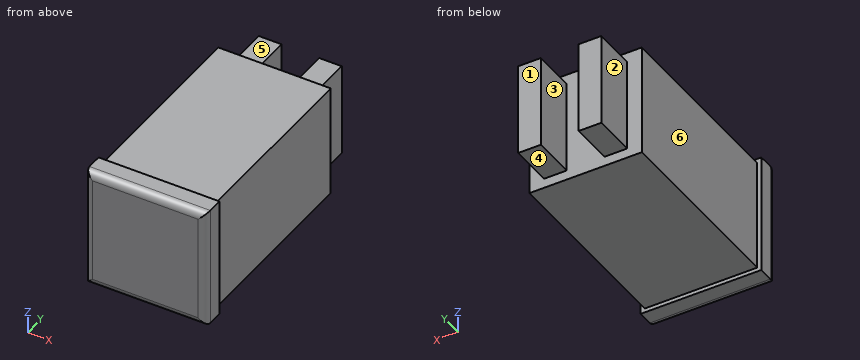
from build123d import *

# Parameters (mm, degrees)
F0_W     = 44.7
F0_H     = 44.7
F0_W_2   = 40.7
F0_H_2   = 40.7
F1_DEPTH = 73
F2_W     = 44.7
F2_H     = 44.7
F2_W_2   = 40.7
F2_H_2   = 40.7
F2_W_3   = 9
F2_H_3   = 37
F3_DEPTH = 3
F4_DEPTH = 20
F0_W_3   = 48
F0_H_3   = 48
F5_DEPTH = 9
F6_R     = 3


with BuildPart() as f1:
    # F0 (on Front) → F1 (new body)
    with BuildSketch(Plane.XZ):
        Rectangle(F0_W, F0_H)
        Rectangle(F0_W_2, F0_H_2, mode=Mode.SUBTRACT)
    extrude(amount=-F1_DEPTH)

    # F2 (on face) → F3 (join)
    with BuildSketch(Plane(origin=(0, 73, 0), x_dir=(-1, 0, 0), z_dir=(0, 1, 0))):
        Rectangle(F2_W, F2_H)
        Rectangle(F2_W_2, F2_H_2, mode=Mode.SUBTRACT)
        Rectangle(F2_W_2, F2_H_2)
        with Locations((-12, 0)):
            Rectangle(F2_W_3, F2_H_3, mode=Mode.SUBTRACT)
        with Locations((12, 0)):
            Rectangle(F2_W_3, F2_H_3, mode=Mode.SUBTRACT)
    extrude(amount=F3_DEPTH)

    # F2 (on face) → F4 (join)
    with BuildSketch(Plane(origin=(0, 73, 0), x_dir=(-1, 0, 0), z_dir=(0, 1, 0))):
        with Locations((-12, 0)):
            Rectangle(F2_W_3, F2_H_3)
        with Locations((12, 0)):
            Rectangle(F2_W_3, F2_H_3)
    extrude(amount=F4_DEPTH)

    # F0 (on Front) → F5 (join)
    with BuildSketch(Plane.XZ):
        Rectangle(F0_W_3, F0_H_3)
        Rectangle(F0_W, F0_H, mode=Mode.SUBTRACT)
        Rectangle(F0_W, F0_H)
        Rectangle(F0_W_2, F0_H_2, mode=Mode.SUBTRACT)
        Rectangle(F0_W_2, F0_H_2)
    extrude(amount=F5_DEPTH)

    # F6
    f6_edges = [f1.edges().sort_by_distance(p)[0] for p in [
        (24, -9, 0),
        (0, -9, 24),
        (-24, -9, 0),
        (0, -9, -24),
    ]]
    fillet(f6_edges, radius=F6_R)


solid = f1.part
Geometry check sheet. Reference: the model listing, model coordinates, mm. Face numbers are marked on the shaded views. A direction names the side the tool comes from. Round coordinates to 2 decimals unless told otherwise and drop trailing zeros. Loops run counter-clockwise (first coordinate to the right, second up) from the corner with the lowest first, then second, coordinate; pieces in that order, holes last. Notation, with made-up numbers: (-35.5, -18.5) -> (19.5, -18.5) arc R23 cw to (19.5, -10.5) -> close; hole circle Ø1 at (-11.5, 66.25). An arc over 180 degrees is marked (long way). Answer as a JSON object with one key per item and string values. Group by question number.
Item 1: Cross-section at A-A, the plane x = -5.5. Record the cut outline in (y, z).
Item 2: Cross-section at B-B, the plane z = -16. Record the cut outline in (x, y), plus the area to 3 significant figures.
Item 3: Set-up check for the marked faces 4, 5 and 6: record each of +Z, -Z, +X, -X, +Y, -Y from which the full face is reachable in a straight line by a thin tool's end or side.
Item 4: Release check for a two-part mould opening along X. For the marked faces 1, 2 and 3 record: pulls with the +X half, pulls with the -X half, needs draft (parallel to the pull), parting line crosses it, or undercut.
Item 5: Cross-section at C-C, the plane y = 26.5. Record the cut outline in (x, z).
Item 6: Thickness scan on line 1 along Y through (x, z) = (-8.5, 4); line 2 along Z through (x, y) = (3, 38). Record the ranges inside material, lowest first.
Item 7: Cross-section at D-D, the plane x = -13.5. Record the cut outline in (y, z), plus the area to 3 significant figures.
Item 8: Depth check by flat-ended pin: pin 1 Ø8 at (x, y) = (16.5, 51) entering from +Z; pin 2 Ø22.5 at (y, z) = (20.5, -9) entering from +X; pin 3 Ø20.5 at (x, z) = (-1.5, 0.5) entering from +Y; pin 4 Ø3 at (y, z) = (73.5, 6.5) entering from -X. Enter the tip coordinate at first touch or a pass-through.
Determined:
{
 "1": {"outline": "(-9, -21) arc R3 ccw to (-6, -24) -> (0, -24) -> (0, -22.35) -> (76, -22.35) -> (76, 22.35) -> (0, 22.35) -> (0, 24) -> (-6, 24) arc R3 ccw to (-9, 21) -> close; hole (0, -20.35) -> (73, -20.35) -> (73, 20.35) -> (0, 20.35) -> close"},
 "2": {"outline": "(-24, -6) arc R3 ccw to (-21, -9) -> (21, -9) arc R3 ccw to (24, -6) -> (24, 0) -> (22.35, 0) -> (22.35, 76) -> (16.5, 76) -> (16.5, 93) -> (7.5, 93) -> (7.5, 76) -> (-7.5, 76) -> (-7.5, 93) -> (-16.5, 93) -> (-16.5, 76) -> (-22.35, 76) -> (-22.35, 0) -> (-24, 0) -> close; hole (-20.35, 0) -> (20.35, 0) -> (20.35, 73) -> (-20.35, 73) -> close", "area": "1,160 mm²"},
 "3": {"face 4": "-Z, +X, -X, +Y", "face 5": "+Z, +X, -X, +Y", "face 6": "+Z, -Z, -X, +Y"},
 "4": {"face 1": "needs draft", "face 2": "pulls with the -X half", "face 3": "undercut"},
 "5": {"outline": "(-22.35, -22.35) -> (22.35, -22.35) -> (22.35, 22.35) -> (-22.35, 22.35) -> close; hole (-20.35, -20.35) -> (20.35, -20.35) -> (20.35, 20.35) -> (-20.35, 20.35) -> close"},
 "6": {"line 1": "y = -9 to 0, 73 to 93", "line 2": "z = -22.35 to -20.35, 20.35 to 22.35"},
 "7": {"outline": "(-9, -21) arc R3 ccw to (-6, -24) -> (0, -24) -> (0, -22.35) -> (76, -22.35) -> (76, -18.5) -> (93, -18.5) -> (93, 18.5) -> (76, 18.5) -> (76, 22.35) -> (0, 22.35) -> (0, 24) -> (-6, 24) arc R3 ccw to (-9, 21) -> close; hole (0, -20.35) -> (73, -20.35) -> (73, 20.35) -> (0, 20.35) -> close", "area": "1,480 mm²"},
 "8": {"pin 1": "stops at z = 22.35", "pin 2": "stops at x = 22.35", "pin 3": "stops at y = 93", "pin 4": "stops at x = -22.35"}
}
